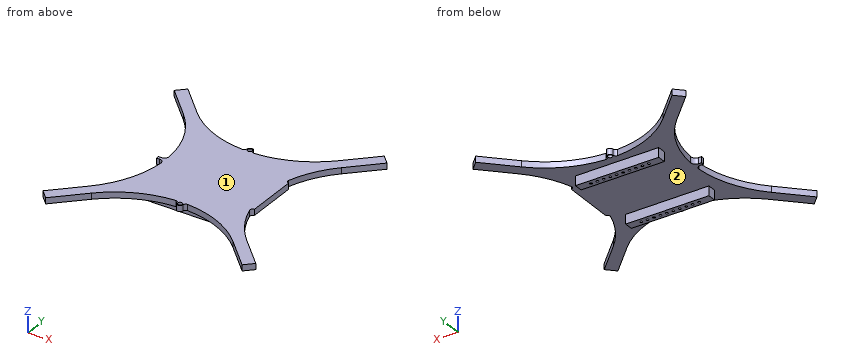
from build123d import *

# Parameters (mm, degrees)
SKETCH1_R           = 0.634780864
BOSS_EXTRUDE1_DEPTH = 1.65
FILLET1_R           = 0.7112
FILLET2_R           = 0.7112
FILLET3_R           = 1.27
SKETCH2_W           = 23
SKETCH2_H           = 2.314
SKETCH2_R           = 0.33
BOSS_EXTRUDE2_DEPTH = 2.6


with BuildPart() as part:
    # Sketch1 → Boss-Extrude1 (new body)
    with BuildSketch(Plane.XY):
        with BuildLine():
            Line((-27.135222714, 29.397964527), (-29.397964527, 27.135222714))
            Line((-29.397964527, 27.135222714), (-21.855060774, 19.592318961))
            ThreePointArc((-21.855060774, 19.592318961), (-15.928204538, 10.7930358), (-13.742710724, 0.41138729))
            Line((-13.742710724, 0.41138729), (-15.908512943, 0.41138729))
            Line((-15.908512943, 0.41138729), (-15.908512943, -0.41138729))
            Line((-15.908512943, -0.41138729), (-13.742710724, -0.41138729))
            ThreePointArc((-13.742710724, -0.41138729), (-15.928204538, -10.7930358), (-21.855060774, -19.592318961))
            Line((-21.855060774, -19.592318961), (-29.397964527, -27.135222714))
            Line((-29.397964527, -27.135222714), (-27.135222714, -29.397964527))
            Line((-27.135222714, -29.397964527), (-19.592318961, -21.855060774))
            ThreePointArc((-19.592318961, -21.855060774), (-10.842511416, -15.949186255), (-0.51885361, -13.744514983))
            ThreePointArc((-0.51885361, -13.744514983), (0, -15.324082887), (0.51885361, -13.744514983))
            ThreePointArc((0.51885361, -13.744514983), (10.842511416, -15.949186255), (19.592318961, -21.855060774))
            Line((19.592318961, -21.855060774), (27.135222714, -29.397964527))
            Line((27.135222714, -29.397964527), (29.397964527, -27.135222714))
            Line((29.397964527, -27.135222714), (21.855060774, -19.592318961))
            ThreePointArc((21.855060774, -19.592318961), (17.437236913, -13.828628501), (14.668755804, -7.114999994))
            Line((14.668755804, -7.114999994), (15.618947426, -7.114999994))
            Line((15.618947426, -7.114999994), (15.618947426, 7.114999994))
            Line((15.618947426, 7.114999994), (14.668755804, 7.114999994))
            ThreePointArc((14.668755804, 7.114999994), (17.437236913, 13.828628501), (21.855060774, 19.592318961))
            Line((21.855060774, 19.592318961), (29.397964527, 27.135222714))
            Line((29.397964527, 27.135222714), (27.135222714, 29.397964527))
            Line((27.135222714, 29.397964527), (19.592318961, 21.855060774))
            ThreePointArc((19.592318961, 21.855060774), (10.842511416, 15.949186255), (0.51885361, 13.744514983))
            ThreePointArc((0.51885361, 13.744514983), (0, 15.324082887), (-0.51885361, 13.744514983))
            ThreePointArc((-0.51885361, 13.744514983), (-10.842511416, 15.949186255), (-19.592318961, 21.855060774))
            Line((-19.592318961, 21.855060774), (-27.135222714, 29.397964527))
        make_face()
        with Locations((0, 14.449082887)):
            Circle(SKETCH1_R, mode=Mode.SUBTRACT)
        with Locations(Location((0, -14.449082887, 0), (0, 0, 180))):
            Circle(SKETCH1_R, mode=Mode.SUBTRACT)
    extrude(amount=BOSS_EXTRUDE1_DEPTH)

    # Fillet1
    fillet1_edges = [part.edges().sort_by_distance(p)[0] for p in [
        (0.51885361, 13.744514983, 0.825),
        (0.51885361, -13.744514983, 0.825),
        (-0.51885361, -13.744514983, 0.825),
        (-0.51885361, 13.744514983, 0.825),
    ]]
    fillet(fillet1_edges, radius=FILLET1_R)

    # Fillet2
    fillet2_edges = [part.edges().sort_by_distance(p)[0] for p in [
        (14.668755804, 7.114999994, 0.825),
        (14.668755804, -7.114999994, 0.825),
    ]]
    fillet(fillet2_edges, radius=FILLET2_R)

    # Fillet3
    fillet3_edges = [part.edges().sort_by_distance(p)[0] for p in [
        (-13.742710724, -0.41138729, 0.825),
        (-13.742710724, 0.41138729, 0.825),
    ]]
    fillet(fillet3_edges, radius=FILLET3_R)

    # Sketch2 → Boss-Extrude2 (add)
    # profile 1 of 2: a face of its own
    with BuildSketch(Plane(origin=(0, 0, 0), x_dir=(-1, 0, 0), z_dir=(0, 0, -1))):
        with Locations((0, 10.385)):
            Rectangle(SKETCH2_W, SKETCH2_H)
        with Locations(Location((-8.002, 10.385, 0), (0, 0, 180))):
            Circle(SKETCH2_R, mode=Mode.SUBTRACT)
        with Locations(Location((-6.224, 10.385, 0), (0, 0, 180))):
            Circle(SKETCH2_R, mode=Mode.SUBTRACT)
        with Locations(Location((-4.446, 10.385, 0), (0, 0, 180))):
            Circle(SKETCH2_R, mode=Mode.SUBTRACT)
        with Locations(Location((-2.668, 10.385, 0), (0, 0, 180))):
            Circle(SKETCH2_R, mode=Mode.SUBTRACT)
        with Locations(Location((-0.89, 10.385, 0), (0, 0, 180))):
            Circle(SKETCH2_R, mode=Mode.SUBTRACT)
        with Locations(Location((0.888, 10.385, 0), (0, 0, 180))):
            Circle(SKETCH2_R, mode=Mode.SUBTRACT)
        with Locations(Location((2.666, 10.385, 0), (0, 0, 180))):
            Circle(SKETCH2_R, mode=Mode.SUBTRACT)
        with Locations(Location((4.444, 10.385, 0), (0, 0, 180))):
            Circle(SKETCH2_R, mode=Mode.SUBTRACT)
        with Locations(Location((6.222, 10.385, 0), (0, 0, 180))):
            Circle(SKETCH2_R, mode=Mode.SUBTRACT)
        with Locations(Location((8, 10.385, 0), (0, 0, 180))):
            Circle(SKETCH2_R, mode=Mode.SUBTRACT)
    # profile 2 of 2: a face of its own
    with BuildSketch(Plane(origin=(0, 0, 0), x_dir=(-1, 0, 0), z_dir=(0, 0, -1))):
        with Locations((0, -10.385)):
            Rectangle(SKETCH2_W, SKETCH2_H)
        with Locations((8, -10.385)):
            Circle(SKETCH2_R, mode=Mode.SUBTRACT)
        with Locations((6.222, -10.385)):
            Circle(SKETCH2_R, mode=Mode.SUBTRACT)
        with Locations((4.444, -10.385)):
            Circle(SKETCH2_R, mode=Mode.SUBTRACT)
        with Locations((2.666, -10.385)):
            Circle(SKETCH2_R, mode=Mode.SUBTRACT)
        with Locations((0.888, -10.385)):
            Circle(SKETCH2_R, mode=Mode.SUBTRACT)
        with Locations((-0.89, -10.385)):
            Circle(SKETCH2_R, mode=Mode.SUBTRACT)
        with Locations((-2.668, -10.385)):
            Circle(SKETCH2_R, mode=Mode.SUBTRACT)
        with Locations((-4.446, -10.385)):
            Circle(SKETCH2_R, mode=Mode.SUBTRACT)
        with Locations((-6.224, -10.385)):
            Circle(SKETCH2_R, mode=Mode.SUBTRACT)
        with Locations((-8.002, -10.385)):
            Circle(SKETCH2_R, mode=Mode.SUBTRACT)
    extrude(amount=BOSS_EXTRUDE2_DEPTH)


solid = part.part
Part model, mm, in its own coordinate system. Face numbers are marked on the shaded views. Give positions to 0.01 mm unless a question says otherwise; leave off trailing zeros. Loops run counter-clockwise (first coordinate to the right, second up) from the corner with the lowest first, then second, coordinate; pieces in that order, holes last.
(1) Pull direction Y, two halves, no side cores. Call the marked faces 1 and 2: pulls with the +Y half, pulls with the -Y half, needs draft (parallel to the pull), parting line crosses it, or undercut.
Return value:
face 1: needs draft
face 2: undercut
(2) Band-saw the part on B-B (y = 17.5). Write the cut outline in (x, z).
Return value:
outline: (-19.97, 0) - (-13.94, 0) - (-13.94, 1.65) - (-19.97, 1.65) - close; (13.94, 0) - (19.97, 0) - (19.97, 1.65) - (13.94, 1.65) - close
(3) Band-saw the part on D-D (y = -5.5). Write the cut outline in (x, z).
Return value:
outline: (-14.29, 0) - (15.62, 0) - (15.62, 1.65) - (-14.29, 1.65) - close
(4) Band-saw the part on C-C (y = -12.5). Write the cut outline in (x, z).
Return value:
outline: (-16.72, 0) - (16.72, 0) - (16.72, 1.65) - (-16.72, 1.65) - close
(5) Band-saw the part on A-A (z = -0.7). Count the separate pieces of the cut face and the enclosed holes in it, and give its area (3 significant figures).
Return value:
separate pieces: 2
enclosed holes: 20
area: 99.6 mm2
(6) Pin check, flat tips, straight feed: pin 1 (1 mm diameter, centred on x = 0, y = 14.45, fed in from +Z); pin 2 (6 mm diameter, centred on x = 2, y = 0, fed in from -Z); pin 3 (1.5 mm diameter, centred on y = -3.5, z = 0, fed in from +X); pin 4 (2.5 mm diameter, centred on y = 10, z = -0.5, fed in from -X). Stop position of each tip, or through.
Return value:
pin 1: passes through
pin 2: stops at z = 0
pin 3: stops at x = 15.62
pin 4: stops at x = -16.08
(7) Drill centre lines: line 1 along Y through (x, z) = (4.5, -1.1); line 2 along Z through (x, y) = (-23.5, -22.5); line 3 along X through (y, z) = (17, 0.15). Where is each one in solid material? Low to high.
Return value:
line 1: y = -11.54 to -10.71, -10.06 to -9.23, 9.23 to 10.06, 10.71 to 11.54
line 2: z = 0 to 1.65
line 3: x = -19.57 to -13.04, 13.04 to 19.57
